For this review, take the finished solid that the model builds, in its own axes (mm). A direction names the side the tool comes from. Give positions to 0.01 mm unless a question says otherwise; leave off trailing zeros. Loops run counter-clockwise (first coordinate to the right, second up) from the corner with the lowest first, then second, coordinate; pieces in that order, holes last. Notation, with made-up numbers: (25, 50.25) - (73, 50.25) arc R31 ccw to (73, 89.25) - close; hole circle Ø9 at (70.25, 43.5). An arc over 180 degrees is marked (long way). Use CSV: the item, a comma, the result in double quotes. Start each with the question number.
1. Wall thickness on line 1 (Y direction, x = -434.5, z = 20); line 2 (Z direction, x = -282, y = -45.5); line 3 (Z direction, x = -132, y = -226.5): over which ranges is each line inside the solid? List them lowest first.
2. Take a section at A-A on y = 152. Give the boundary of the cut face in (x, z).
3. For faces 4 (the cylindrical face through (44.7, -209.9, 6.3)), 5 (the flat face through (-292, 247, 25.4)), 6 (the flat face through (-190, -285.16, 13)), 7 (the flat face through (-283, -30, 25.4)), 8 (the flat face through (-440, -172, 12.7)), list the 3-axis set-ups (+Z, -Z, +X, -X, +Y, -Y) from which the entire face can be reached by the end or side of a thin tool; tool diameter is ignored.
4. Mouldability with a two-part tool opening along Z and no side actions: class faces 1 (the flat face through (-432, -139, 25.4)), 2 (the flat face through (-134.06, 86.16, 12.52)), 3 (the flat face through (-140.35, 110.77, 31.66)) as pulls with the +Z half, pulls with the -Z half, needs draft (parallel to the pull), parting line crosses it, or undercut.
5. Take a section at B-B on y = 82. Give the boundary of the cut face in (x, z).
6. For pin 1 (4 mm diameter, centred on x = -220.5, y = -224.5, fed in from +Z); pin 2 (12.5 mm diameter, centred on x = -269.5, z = 11, fed in from +Y); pin 3 (14 mm diameter, centred on x = -465.5, y = -252.5, fed in from +Z), all flat-tipped, find the tip position at first contact; note any pin that passes through.
7. Take a section at C-C on y = -115. Give the boundary of the cut face in (x, z).
```python
from build123d import *

# Parameters (mm, degrees)
SKETCH1_W            = 600
SKETCH1_H            = 600
BOSS_EXTRUDE1_DEPTH  = 76.2
BOSS_EXTRUDE2_DEPTH  = 25.4
BOSS_EXTRUDE3_START  = 25.4
BOSS_EXTRUDE3_DEPTH  = 12.7
BOSS_EXTRUDE4_DEPTH  = 25.4
BOSS_EXTRUDE5_START  = 25.4
BOSS_EXTRUDE5_DEPTH  = 12.7
BOSS_EXTRUDE6_DEPTH  = 25.4
SKETCH1_42_W         = 482.6
SKETCH1_42_H         = 12.7
SKETCH1_42_W_2       = 469.9
SKETCH1_42_W_3       = 508
BOSS_EXTRUDE7_DEPTH  = 25.4
BOSS_EXTRUDE8_DEPTH  = 12.7
BOSS_EXTRUDE9_START  = 25.4
BOSS_EXTRUDE9_DEPTH  = 12.7
BOSS_EXTRUDE10_DEPTH = 25.4


with BuildPart() as part:
    # Sketch1 → Boss-Extrude1 (new body)
    with BuildSketch(Plane.XY):
        with Locations((-225.240056073, 6.540000857)):
            Rectangle(SKETCH1_W, SKETCH1_H)
    extrude(amount=-BOSS_EXTRUDE1_DEPTH)

    # Sketch1_22 → Boss-Extrude2 (add)
    with BuildSketch(Plane.XY):
        Polygon((-525.240056073, 242.984461231), (-525.240056073, 255.740000857), (-49.879871206, 211.234703059), (-51.063723483, 198.590000857), align=None)
    extrude(amount=BOSS_EXTRUDE2_DEPTH)

    # Sketch1_23 → Boss-Extrude3 (add)
    with BuildSketch(Plane.XY.offset(BOSS_EXTRUDE3_START)):
        Polygon((-525.240056073, 242.984461231), (-57.386074584, 199.181926995), (-53.834517754, 237.116033602), (-521.688499243, 280.918567838), align=None)
    extrude(amount=BOSS_EXTRUDE3_DEPTH)

    # Sketch1_36 → Boss-Extrude4 (add)
    with BuildSketch(Plane.XY):
        Polygon((-342.440287545, 17.406237518), (74.759943927, 128.740000857), (71.744479474, 141.079727937), (-345.714809996, 29.676832561), align=None)
    extrude(amount=BOSS_EXTRUDE4_DEPTH)

    # Sketch1_38 → Boss-Extrude5 (add)
    with BuildSketch(Plane.XY.offset(BOSS_EXTRUDE5_START)):
        Polygon((-342.440287545, 17.406237518), (74.759943927, 128.740000857), (65.713550566, 165.759182097), (-352.263854899, 54.218022648), align=None)
    extrude(amount=BOSS_EXTRUDE5_DEPTH)

    # Sketch1_39 → Boss-Extrude6 (add)
    with BuildSketch(Plane.XY):
        with BuildLine():
            Line((-515.232510143, 14.731286418), (-511.049397451, 39.784461231))
            add(Edge.make_bspline(
                [(-511.049397451, 39.784461231), (-491.91342743, 29.210221806), (-458.77856372, 19.531721492), (-416.625986292, 3.959066392), (-383.903580076, -6.249374557), (-350.315397205, -13.252889549), (-315.502078412, -21.570378936), (-279.518469533, -27.808056985), (-243.831298859, -34.151990356), (-199.456462469, -34.752149035), (-135.713837898, -30.00036949), (-83.078004242, -31.661348956), (-53.461097288, -19.3009415)],
                knots=[0, 0, 0, 0, 0.138195141, 0.220153512, 0.28706639, 0.356885041, 0.439197272, 0.515633138, 0.590194642, 0.670343679, 0.797980141, 1, 1, 1, 1], degree=3))
            Line((-53.461097288, -19.3009415), (-53.461097288, -44.7009415))
            add(Edge.make_bspline(
                [(-515.232510143, 14.731286418), (-492.287448082, 7.361196537), (-460.683716745, -0.781157172), (-419.974441586, -13.502513213), (-388.83188488, -22.419811825), (-355.455504677, -31.276728095), (-317.590964539, -38.781286591), (-279.774049612, -45.52299243), (-241.592265326, -48.592909593), (-194.728275521, -49.903260595), (-132.907153847, -52.623676823), (-81.911313969, -45.613021801), (-53.461097288, -44.7009415)],
                knots=[0, 0, 0, 0, 0.153828341, 0.208264646, 0.272296669, 0.360672756, 0.428620212, 0.51872685, 0.605764862, 0.672841047, 0.818182432, 1, 1, 1, 1], degree=3))
        make_face()
    extrude(amount=BOSS_EXTRUDE6_DEPTH)

    # Sketch1_42 → Boss-Extrude7 (add)
    with BuildSketch(Plane.XY):
        with Locations((-199.186590665, -202.053329244)):
            Rectangle(SKETCH1_42_W, SKETCH1_42_H)
        with Locations((-207.36885806, -227.48194535)):
            Rectangle(SKETCH1_42_W_2, SKETCH1_42_H)
        with Locations((-186.486590665, -278.810327036)):
            Rectangle(SKETCH1_42_W_3, SKETCH1_42_H)
    extrude(amount=BOSS_EXTRUDE7_DEPTH)

    # Sketch1_43 → Boss-Extrude8 (add)
    with BuildSketch(Plane.XY):
        Polygon((-504.347920448, -169.394549915), (-503.794481482, -163.068713582), (-377.277754824, -174.137492911), (-377.831193791, -180.463329244), align=None)
        Polygon((-377.681842187, -251.203045623), (-504.198568844, -240.134266294), (-504.752007811, -246.460102627), (-378.235281153, -257.528881956), align=None)
        with BuildLine():
            Line((55.52114194, -195.703329244), (50.469758046, -195.703329244))
            ThreePointArc((50.469758046, -195.703329244), (44.509786376, -210.09197368), (30.12114194, -216.05194535))
            Line((30.12114194, -216.05194535), (30.12114194, -221.103329244))
            ThreePointArc((30.12114194, -221.103329244), (48.081654182, -213.663841486), (55.52114194, -195.703329244))
        make_face()
    extrude(amount=BOSS_EXTRUDE8_DEPTH)



with BuildPart() as body_2:
    # Sketch1_46 → Boss-Extrude9 (new body)
    with BuildSketch(Plane.XY.offset(BOSS_EXTRUDE9_START)):
        Polygon((74.759943927, -71.628181651), (69.260201501, -33.927215705), (-427.135850118, -106.340490986), (-421.636107692, -144.041456932), align=None)
    extrude(amount=BOSS_EXTRUDE9_DEPTH)


with BuildPart() as part_1:
    add(part.part)

    add(body_2.part)  # Boss-Extrude10 merges body 2
    # Sketch1_47 → Boss-Extrude10 (add)
    with BuildSketch(Plane.XY):
        Polygon((-440.486590665, -146.791328145), (-421.636107692, -144.041456932), (-423.469355167, -131.474468283), (-442.31983814, -134.224339496), align=None)
        Polygon((-421.636107692, -144.041456932), (74.759943927, -71.628181651), (72.926696452, -59.061193002), (-423.469355167, -131.474468283), align=None)
    extrude(amount=BOSS_EXTRUDE10_DEPTH)


solid = part_1.part
```
Check result:
1,line 1,"y = -285.16 to -272.46, -233.83 to -221.13, -208.4 to -195.7, -145.92 to -133.08, -8.97 to 10.54, 234.49 to 247.24"
1,line 2,"z = -76.2 to 0"
1,line 3,"z = -76.2 to 25.4"
2,outline,"(-525.24, -76.2) - (74.76, -76.2) - (74.76, 0) - (-525.24, 0) - close; (14.15, 25.4) - (69.08, 25.4) - (69.08, 38.1) - (14.15, 38.1) - close"
3,face 4,"+Z"
3,face 5,"+X, +Y"
3,face 6,"+Z, +X, -X, -Y"
3,face 7,"+Z, -X"
3,face 8,"+Z, +X, -X"
4,face 1,"pulls with the +Z half"
4,face 2,"undercut"
4,face 3,"needs draft"
5,outline,"(-525.24, -76.2) - (74.76, -76.2) - (74.76, 0) - (-100.39, 0) - (-100.39, 38.1) - (-248.16, 38.1) - (-248.16, 25.4) - (-149.64, 25.4) - (-149.64, 0) - (-525.24, 0) - close"
6,pin 1,"stops at z = 25.4"
6,pin 2,"stops at y = 232.38"
6,pin 3,"stops at z = 12.7"
7,outline,"(-525.24, -76.2) - (74.76, -76.2) - (74.76, 0) - (-222.56, 0) - (-222.56, 38.1) - (-425.87, 38.1) - (-425.87, 25.4) - (-310.54, 25.4) - (-310.54, 0) - (-525.24, 0) - close"
